Input: part model. Units: mm. Frame: model coordinates. Face numbers are marked on the shaded views. Round coordinates to 2 decimals unless told otherwise and drop trailing zeros. Loops run counter-clockwise (first coordinate to the right, second up) from the corner with the lowest first, then second, coordinate; pieces in that order, holes last. Notation, with made-up numbers: (-10, -24) - (36, -24) arc R9 cw to (36, -15) - close; hole circle Ø3 at (67, 72). An arc over 180 degrees is marked (long way). One line per question, with ' | ' between items. Start each with the question number.
Item 1: Draft query along Z for the marked faces 1, 2, 3 and 4. Return one class per face: pulls with the +Z half, pulls with the -Z half, needs draft (parallel to the pull), parting line crosses it, or undercut.
Item 2: Section B-B, the plane z = 0. Return loops of the section in (x, y).
Item 3: First-contact query: pin 1 (5 mm diameter, centred on x = 34, y = 212.5, fed in from +Z); pin 2 (4 mm diameter, centred on x = -32, y = 105.5, fed in from -Z); pin 3 (4 mm diameter, centred on y = 210, z = 94.5, fed in from -X). Flat tips, straight axial feed; report the tip coordinate or a pass-through.
Item 4: Material intervals for line 1 along Y through (x, z) = (1, -13); line 2 along Z through (x, y) = (32.5, 120.5); line 3 along Z through (x, y) = (70, 60.5), sorted ascending.
Item 5: Section C-C, the plane y = 98. Return loops of the section in (x, z), plus the area to 3 significant figures.
Item 6: Section A-A, the plane x = 0. Return loops of the section in (y, z).
Item 7: Section D-D, the plane y = 66. Return loops of the section in (x, z), plus the area to 3 significant figures.
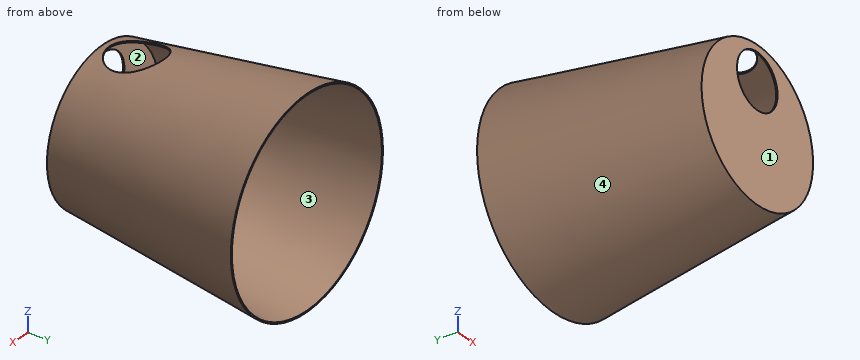
```python
from build123d import *

# Parameters (mm, degrees)
SHELL_1_T           = -2
SKETCH_2_R          = 40
CUT_EXTRUDE_1_DEPTH = 368.423461417
SKETCH_3_R          = 40
CUT_EXTRUDE_7_DEPTH = 10


with BuildPart() as part:
    # 草圖1 → 旋轉1 (revolve)
    with BuildSketch(Plane.XY):
        Polygon((-150, 300), (-110, 0), (0, 0), (0, 300), align=None)
    revolve(axis=Axis((0, 300, 0), (0, -1, 0)))

    # 薄殼1
    shell_1_openings = [part.faces().sort_by_distance(p)[0] for p in [
        (0, 300, 0),
    ]]
    offset(amount=SHELL_1_T, openings=shell_1_openings, kind=Kind.INTERSECTION)

    # 草圖2 → 除料-伸長1 (cut, through all)
    with BuildSketch(Plane.XY):
        with Locations(Location((0, 50, 0), (0, 0, 223.831442038))):
            Circle(SKETCH_2_R)
    extrude(amount=CUT_EXTRUDE_1_DEPTH, mode=Mode.SUBTRACT)

    # 草圖3 → 除料-伸長7 (cut)
    with BuildSketch(Plane(origin=(0, 0, 0), x_dir=(1, 0, 0), z_dir=(0, 1, 0))):
        with Locations((0, -60)):
            Circle(SKETCH_3_R)
    extrude(amount=CUT_EXTRUDE_7_DEPTH, mode=Mode.SUBTRACT)


solid = part.part
```
Return value:
1) face 1: needs draft | face 2: undercut | face 3: undercut | face 4: parting line crosses it
2) outline: (-150, 300) - (-110, 0) - (110, 0) - (150, 300) - (147.98, 300) - (108.25, 2) - (-108.25, 2) - (-147.98, 300) - close
3) pin 1: z = 134.79 | pin 2: z = -120.46 | pin 3: x = -102.45
4) line 1: 0 to 2 | line 2: -121.81 to -119.72, 119.72 to 121.81 | line 3: -95.08 to -92.56, 92.56 to 95.08
5) outline: circle Ø246.13 at (0, 0); hole circle Ø242.1 at (0, 0) | area: 1,550 mm2
6) outline: (0, -110) - (300, -150) - (300, -147.98) - (2, -108.25) - (2, 20) - (0, 20) - close; (0, 100) - (2, 100) - (2, 108.25) - (10, 109.32) - (10, 111.33) - (0, 110) - close; (90, 119.98) - (300, 147.98) - (300, 150) - (90, 122) - close
7) outline: (-36.66, 110.88) - (-36.66, 113) arc R118.8 ccw (long way) to (36.66, 113) - (36.66, 110.88) arc R116.78 cw (long way) to start | area: 1,340 mm2
